from build123d import *

# Parameters (mm, degrees)
SKETCH_1_R             = 4
SKETCH_1_R_2           = 2
SKETCH_1_R_3           = 5
SKETCH_1_R_4           = 1.5
SM_BASE_FLANGE_1_DEPTH = 3


# Sheet-metal steps are written as plain solids
with BuildPart() as part:
    # Sketch 1 → 基体-法兰1 (new body)
    with BuildSketch(Plane(origin=(0, 0, 0), x_dir=(1, 0, 0), z_dir=(0, 1, 0))):
        with BuildLine():
            Line((22, 200), (22, 0))
            ThreePointArc((22, 0), (0, -22), (-22, 0))
            Line((-22, 0), (-22, 200))
            ThreePointArc((-22, 200), (0, 222), (22, 200))
        make_face()
        with Locations(Location((0, 0, 0), (0, 0, 270))):
            Circle(SKETCH_1_R, mode=Mode.SUBTRACT)
        with Locations(Location((-10, 35, 0), (0, 0, 270))):
            Circle(SKETCH_1_R_2, mode=Mode.SUBTRACT)
        with Locations(Location((10, 35, 0), (0, 0, 270))):
            Circle(SKETCH_1_R_2, mode=Mode.SUBTRACT)
        with Locations(Location((-10, 135, 0), (0, 0, 270))):
            Circle(SKETCH_1_R_2, mode=Mode.SUBTRACT)
        with Locations(Location((10, 135, 0), (0, 0, 270))):
            Circle(SKETCH_1_R_2, mode=Mode.SUBTRACT)
        with Locations(Location((0, 200, 0), (0, 0, 270))):
            Circle(SKETCH_1_R_3, mode=Mode.SUBTRACT)
        with Locations(Location((0, 215, 0), (0, 0, 270))):
            Circle(SKETCH_1_R_4, mode=Mode.SUBTRACT)
        with Locations(Location((15, 200, 0), (0, 0, 270))):
            Circle(SKETCH_1_R_4, mode=Mode.SUBTRACT)
        with Locations(Location((0, 185, 0), (0, 0, 270))):
            Circle(SKETCH_1_R_4, mode=Mode.SUBTRACT)
        with Locations(Location((-15, 200, 0), (0, 0, 270))):
            Circle(SKETCH_1_R_4, mode=Mode.SUBTRACT)
        with Locations(Location((0, 15, 0), (0, 0, 270))):
            Circle(SKETCH_1_R_2, mode=Mode.SUBTRACT)
        with Locations(Location((15, 0, 0), (0, 0, 270))):
            Circle(SKETCH_1_R_2, mode=Mode.SUBTRACT)
        with Locations(Location((0, -15, 0), (0, 0, 270))):
            Circle(SKETCH_1_R_2, mode=Mode.SUBTRACT)
        with Locations(Location((-15, 0, 0), (0, 0, 270))):
            Circle(SKETCH_1_R_2, mode=Mode.SUBTRACT)
    extrude(amount=-SM_BASE_FLANGE_1_DEPTH)


solid = part.part
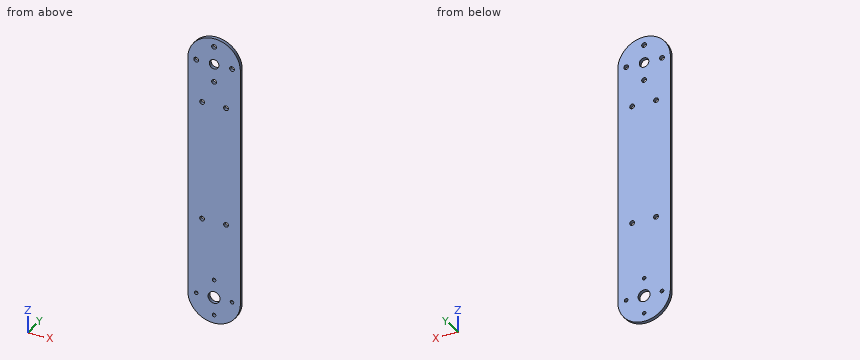
Verification items for the finished model (mm, model axes). Coordinates: 2 decimals unless noted, no trailing zeros. Loops run counter-clockwise (first coordinate to the right, second up) from the corner with the lowest first, then second, coordinate; pieces in that order, holes last. Notation, with made-up numbers: (-3.5, 32.5) -> (17.5, 32.5) arc R14 ccw to (17.5, 48.5) -> close; hole circle Ø9 at (61.25, 47.5). An arc over 180 degrees is marked (long way). Answer as a JSON object with one key per item and string values. Group by question number.
Item 1: Sectioned sample at B-B on y = -1.3. State how many separate pieces and enclosed holes the cut face has, plus the area to 3 significant figures.
Item 2: Sectioned sample at C-C on x = 10. Record the boundary of the cut face in (y, z), plus the area to 3 significant figures.
Item 3: Sectioned sample at D-D on z = 15. Record the boundary of the cut face in (x, y), plus the area to 3 significant figures.
Item 4: Depth check by flat-ended pin: pin 1 (5 mm diameter, centred on x = 15, z = 0, fed in from +Y); pin 2 (3.5 mm diameter, centred on x = 0, z = -15, fed in from +Y). Enter the tip coordinate at first touch or a pass-through.
Item 5: Scan lines: probe 1 along X at (y, z) = (-1.3, -200); probe 2 along X at (y, z) = (-0.85, 0); probe 3 along X at (y, z) = (-0.7, -135). Record each from-to range of solid material in increasing order.
Item 6: Sectioned sample at A-A on z = -35. Record the boundary of the cut face in (x, y), plus the area to 3 significant figures.
Evaluation:
{
 "1": {"separate pieces": "1", "enclosed holes": "14", "area": "10,100 mm²"},
 "2": {"outline": "(-3, -219.6) -> (0, -219.6) -> (0, -137) -> (-3, -137) -> close; (-3, -133) -> (0, -133) -> (0, -37) -> (-3, -37) -> close; (-3, -33) -> (0, -33) -> (0, 19.6) -> (-3, 19.6) -> close", "area": "694 mm²"},
 "3": {"outline": "(-16.09, -3) -> (-2, -3) -> (-2, 0) -> (-16.09, 0) -> close; (2, -3) -> (16.09, -3) -> (16.09, 0) -> (2, 0) -> close", "area": "84.6 mm²"},
 "4": {"pin 1": "stops at y = 0", "pin 2": "passes through"},
 "5": {"probe 1": "x = -22 to -16.5, -13.5 to -5, 5 to 13.5, 16.5 to 22", "probe 2": "x = -22 to -17, -13 to -4, 4 to 13, 17 to 22", "probe 3": "x = -22 to -12, -8 to 8, 12 to 22"},
 "6": {"outline": "(-22, -3) -> (-12, -3) -> (-12, 0) -> (-22, 0) -> close; (-8, -3) -> (8, -3) -> (8, 0) -> (-8, 0) -> close; (12, -3) -> (22, -3) -> (22, 0) -> (12, 0) -> close", "area": "108 mm²"}
}
